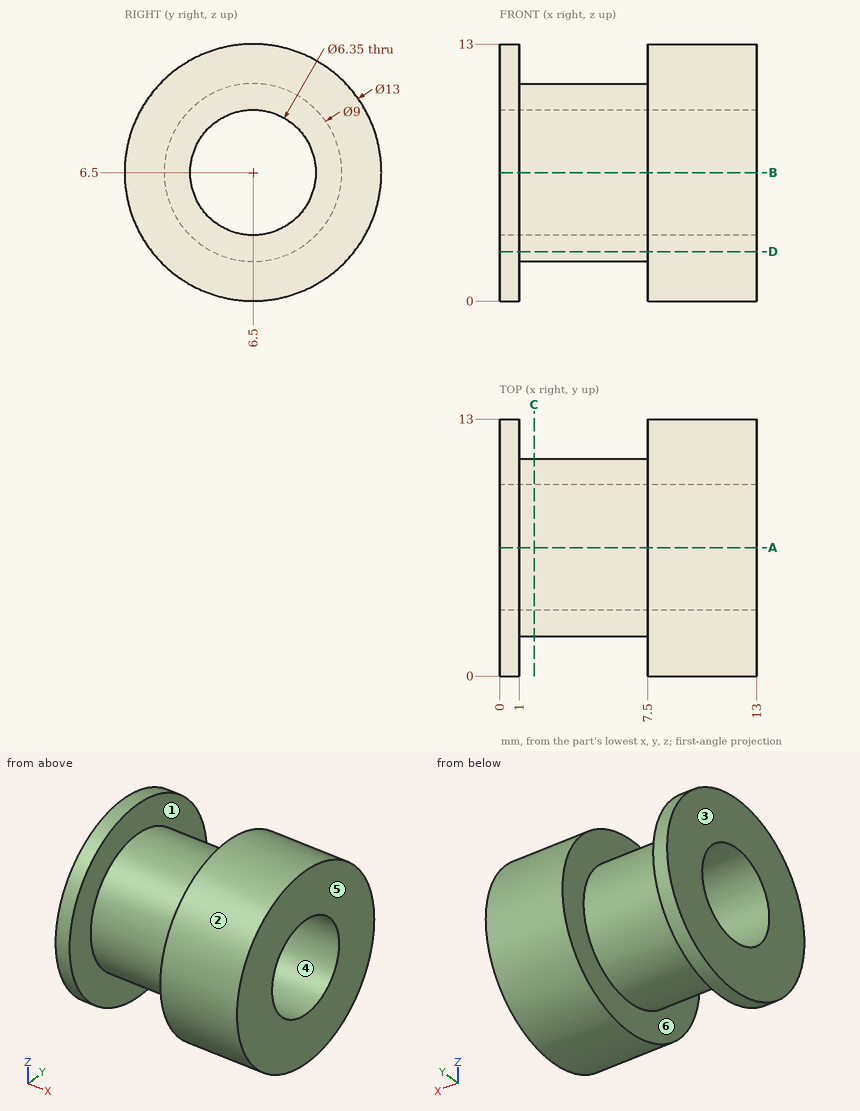
The drawing under review shows one solid part. Ordinate dimensions are in mm from its lowest x, y, z. A direction names the side the tool comes from. Coordinates: 2 decimals unless noted, no trailing zeros. Order: outer loops, then holes, each group sorted by start corner. A loop starts at its lowest first (then second) coordinate and runs counter-clockwise, first axis right, second up. Notation, with made-up numbers: (44.25, -34) -> (59.25, -34) arc R18 cw to (59.25, -11) -> close; hole circle Ø9 at (30, 31.25). An arc over 180 degrees is marked (long way). Answer as CSV lines item,"result".
Q1. We need section A-A (y = 6.5). State the section outline as (x, z) points (3 decimals), plus the area to 4 significant figures.
Model answer:
outline,"(0, 0) -> (1, 0) -> (1, 2) -> (7.5, 2) -> (7.5, 0) -> (13, 0) -> (13, 3.325) -> (0, 3.325) -> close; (0, 9.675) -> (13, 9.675) -> (13, 13) -> (7.5, 13) -> (7.5, 11) -> (1, 11) -> (1, 13) -> (0, 13) -> close"
area,"60.45 mm2"
Q2. We need section D-D (z = 2.5). State the section outline as (x, y) points, plus the area to 3 significant figures.
Model answer:
outline,"(0, 1.38) -> (1, 1.38) -> (1, 4.44) -> (7.5, 4.44) -> (7.5, 1.38) -> (13, 1.38) -> (13, 11.62) -> (7.5, 11.62) -> (7.5, 8.56) -> (1, 8.56) -> (1, 11.62) -> (0, 11.62) -> close"
area,"93.4 mm2"
Q3. For the marked faces 1 and 2, list the 3-axis set-ups (+Z, -Z, +X, -X, +Y, -Y) from which the entire face can be reached by the end or side of a thin tool; tool diameter is ignored.
Model answer:
face 1,"none"
face 2,"+X, -X"
Q4. Clearance check with flat-ended pins moving along their axes: pin 1 Ø5 at (x, z) = (4, 9.5) entering from -Y; pin 2 Ø6.5 at (y, z) = (6, 9.5) entering from -X; pin 3 Ø1 at (x, z) = (5, 11) entering from +Y; pin 4 Ø1 at (x, y) = (3, 5.5) entering from +Z. State where each tip first meets the part, or that it passes through.
Model answer:
pin 1,"stops at y = 2.03"
pin 2,"stops at x = 0"
pin 3,"stops at y = 8.56"
pin 4,"stops at z = 10.97"
Q5. We need section C-C (x = 1.75). State the section outline as (y, z) points (3 decimals), plus the area to 3 significant figures.
Model answer:
outline,"circle Ø9 at (6.5, 6.5); hole circle Ø6.35 at (6.5, 6.5)"
area,"31.9 mm2"
Q6. Draft analysis for pull direction X (two halves, no side actions). For the marked faces 3, 4, 5 and 6, state which applies: released by +X, released by -X, zero draft, split by the parting line, or undercut.
Model answer:
face 3,"released by -X"
face 4,"zero draft"
face 5,"released by +X"
face 6,"undercut"
Q7. Wall thickness on line 1 along X through (y, z) = (4, 2.25); line 2 along Z through (x, y) = (5.5, 7.5); line 3 along Y through (x, z) = (2.25, 8.75): over which ranges is each line inside the solid? List them lowest first. Write a range as [from, to].
Model answer:
line 1,"x = [0, 1], [7.5, 13]"
line 2,"z = [2.11, 3.49], [9.51, 10.89]"
line 3,"y = [2.6, 4.26], [8.74, 10.4]"
